CAD build for the part. Positions are in the model's coordinates, mm. Face numbers are marked on the shaded views. A direction names the side the tool comes from. Round coordinates to 2 decimals unless told otherwise and drop trailing zeros. Loops run counter-clockwise (first coordinate to the right, second up) from the corner with the lowest first, then second, coordinate; pieces in that order, holes last.
from build123d import *

# Parameters (mm, degrees)
SKETCH_1_W          = 96
SKETCH_1_H          = 113
EXTRUDE_1_DEPTH     = 50
SKETCH_2_W          = 67
SKETCH_2_H          = 113
CUT_EXTRUDE_1_DEPTH = 10
SKETCH_3_W          = 60
SKETCH_3_H          = 113
SKETCH_3_W_2        = 30
CUT_EXTRUDE_2_DEPTH = 38
SKETCH_4_W          = 80
SKETCH_4_H          = 15
CUT_EXTRUDE_3_DEPTH = 2


with BuildPart() as part:
    # Эскиз1 → Бобышка-Вытянуть1 (new body)
    with BuildSketch(Plane(origin=(0, 0, 0), x_dir=(1, 0, 0), z_dir=(0, 1, 0))):
        with Locations((48, 56.5)):
            Rectangle(SKETCH_1_W, SKETCH_1_H)
    extrude(amount=EXTRUDE_1_DEPTH)

    # Эскиз2 → Вырез-Вытянуть1 (cut)
    with BuildSketch(Plane(origin=(0, 50, 0), x_dir=(1, 0, 0), z_dir=(0, 1, 0))):
        with Locations((48, 56.5)):
            Rectangle(SKETCH_2_W, SKETCH_2_H)
    extrude(amount=-CUT_EXTRUDE_1_DEPTH, mode=Mode.SUBTRACT)

    # Эскиз3 → Вырез-Вытянуть2 (cut)
    with BuildSketch(Plane.XZ):
        with Locations((32, -56.5)):
            Rectangle(SKETCH_3_W, SKETCH_3_H)
        with Locations((79, -56.5)):
            Rectangle(SKETCH_3_W_2, SKETCH_3_H)
    extrude(amount=-CUT_EXTRUDE_2_DEPTH, mode=Mode.SUBTRACT)

    # Эскиз4 → Вырез-Вытянуть3 (cut)
    with BuildSketch(Plane.ZY):
        with Locations((-66, 28.5)):
            Rectangle(SKETCH_4_W, SKETCH_4_H)
    extrude(amount=-CUT_EXTRUDE_3_DEPTH, mode=Mode.SUBTRACT)


solid = part.part
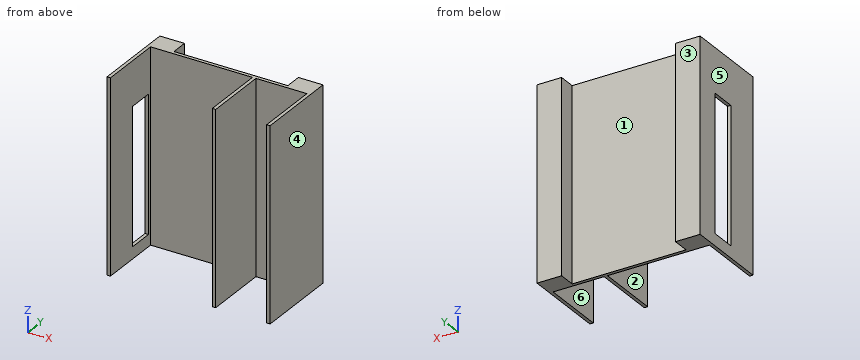
Item 1: Wall check: L1, parallel to X at y = 12.5, z = -96; L2, parallel to X at y = 44, z = -18.5; L3, parallel to Y at x = 71.5, z = -17. Give the ranges that are in metal, low to high.
Verdict:
L1: x = 0 to 2, 62 to 64, 94 to 96
L2: x = 0 to 14.5, 81.5 to 96
L3: y = 38 to 40
Item 2: Cut at C-C (y = 30.5). List the corners of the cut face in (x, z), plus the area to 3 significant figures.
Verdict:
outline: (0, -113) - (2, -113) - (2, -106) - (0, -106) - close; (0, -26) - (2, -26) - (2, 0) - (0, 0) - close; (62, -113) - (64, -113) - (64, 0) - (62, 0) - close; (94, -113) - (96, -113) - (96, 0) - (94, 0) - close
area: 518 mm2
Item 3: Flat gauge pins, fed straight in: P1, Ø2, axis at x = 1.5, y = 29.5, coming from the +Z side; P2, Ø5, axis at y = 29.5, z = -51.5, coming from the -X side; P3, Ø9, axis at x = 76.5, z = -68, coming from the -Y side; P4, Ø8, axis at x = 32.5, z = -78, coming from the +Y side. Where does each tip first touch, or does it go through?
Verdict:
P1: stops at z = 0
P2: stops at x = 62
P3: stops at y = 38
P4: stops at y = 40
Item 4: Mould opens along X. For the marked faces 4, 5 and 6 say: released by +X, released by -X, zero draft, split by the parting line, or undercut.
Verdict:
face 4: released by +X
face 5: released by -X
face 6: undercut
Item 5: Cut at A-A (y = 4). List the corners of the cut face in (x, z), plus the area to 3 significant figures.
Verdict:
outline: (0, -113) - (2, -113) - (2, 0) - (0, 0) - close; (62, -113) - (64, -113) - (64, 0) - (62, 0) - close; (94, -113) - (96, -113) - (96, 0) - (94, 0) - close
area: 678 mm2
Item 6: Cut at D-D (y = 46.5). List the corners of the cut face in (x, z), plus the area to 3 significant figures.
Verdict:
outline: (0, -113) - (14.5, -113) - (14.5, 0) - (0, 0) - close; (81.5, -113) - (96, -113) - (96, 0) - (81.5, 0) - close
area: 3,280 mm2
Item 7: 3-axis set-ups, long thin cutter, end or side, ignore diameter. For the marked faces 1, 2 and 3: which of +Z, -Z, +X, -X, +Y, -Y reach the whole face in a straight line?
Verdict:
face 1: +Z, -Z, +Y
face 2: +Z, -Z, -Y
face 3: +Z, -Z, +X, -X, +Y
Item 8: Cut at B-B (z = -104). List the corners of the cut face in (x, y).
Verdict:
outline: (0, 0) - (2, 0) - (2, 21) - (0, 21) - close; (0, 36) - (2, 36) - (2, 38) - (62, 38) - (62, 0) - (64, 0) - (64, 38) - (94, 38) - (94, 0) - (96, 0) - (96, 50) - (81.5, 50) - (81.5, 40) - (14.5, 40) - (14.5, 50) - (0, 50) - close
